Design review of the part built by this model. Coordinates are the model's own, in mm. A direction names the side the tool comes from. Coordinates: 2 decimals unless noted, no trailing zeros. Loops run counter-clockwise (first coordinate to the right, second up) from the corner with the lowest first, then second, coordinate; pieces in that order, holes last. Notation, with made-up numbers: (-33.5, 83) -> (-0.5, 83) arc R26 ccw to (-0.5, 106) -> close; hole circle Ø10 at (10.25, 23.5). An arc over 180 degrees is marked (long way). Use a Markdown table: item, result. Add a question column.
Q1. Take a section at B-B on x = 5. Write out the cut boundary in (y, z).
Q2. Clearance check with a flat-ended pin moving along its axis: pin 1 Ø2 at (x, y) = (134.5, 5) entering from -Z. State where the tip first meets the part, or that it passes through.
Q3. Draft analysis for pull direction Z (two halves, no side actions). For faces 1 (the face through (37, 5, 5)), 2 (the face through (5.766, 4.93, 28.847)), 3 (the face through (84, 5, 160)), state which applies: pulls with the +Z half, pulls with the -Z half, needs draft (parallel to the pull), parting line crosses it, or undercut.
Q4. For faces 4 (the face through (133, 5, 5)), 5 (the face through (84, 10, 79)), 6 (the face through (38.55, 5, 13)), list the 3-axis set-ups (+Z, -Z, +X, -X, +Y, -Y) from which the entire face can be reached by the end or side of a thin tool; tool diameter is ignored.
Q5. Take a section at A-A on z = 27. Write out the cut boundary in (x, y), plus the area to 3 significant figures.
Q6. For probe 1 along Z at (x, y) = (165, 7.5); probe 2 along X at (y, z) = (3.75, 133); probe 3 along X at (y, z) = (9.25, 13.5), list the stretches that pass through material, from the lowest coordinate up.
from build123d import *

# Parameters (mm, degrees)
SKETCH1_W               = 170
SKETCH1_H               = 10
BOSS_EXTRUDE1_DEPTH     = 160
ESQUISSE1_R             = 2
ENL_V_MAT_EXTRU_2_DEPTH = 10
ENL_V_MAT_EXTRU_3_DEPTH = 10


with BuildPart() as part:
    # Sketch1 → Boss-Extrude1 (new body)
    with BuildSketch(Plane.XY):
        with Locations((85, 5)):
            Rectangle(SKETCH1_W, SKETCH1_H)
    extrude(amount=BOSS_EXTRUDE1_DEPTH)

    # Esquisse1 → Enlèv. mat.-Extru.2 (cut)
    with BuildSketch(Plane.XZ):
        with Locations(Location((5, 133, 0), (0, 0, 270))):
            Circle(ESQUISSE1_R)
        with Locations(Location((5, 27, 0), (0, 0, 90))):
            Circle(ESQUISSE1_R)
        with Locations(Location((165, 27, 0), (0, 0, 270))):
            Circle(ESQUISSE1_R)
        with Locations(Location((165, 133, 0), (0, 0, 90))):
            Circle(ESQUISSE1_R)
    extrude(amount=-ENL_V_MAT_EXTRU_2_DEPTH, mode=Mode.SUBTRACT)

    # Esquisse2 → Enlèv. mat.-Extru.3 (cut)
    with BuildSketch(Plane(origin=(0, 0, 0), x_dir=(-1, 0, 0), z_dir=(0, -1, 0))):
        Polygon((-133, -10), (-133, 0), (-137, 0), (-137, -10), (-138.55, -10), (-138.55, -15.5), (-137, -15.5), (-137, -21.5), (-133, -21.5), (-133, -15.5), (-131.45, -15.5), (-131.45, -10), align=None)
        Polygon((-33, -10), (-33, 0), (-37, 0), (-37, -10), (-38.55, -10), (-38.55, -15.5), (-37, -15.5), (-37, -21.5), (-33, -21.5), (-33, -15.5), (-31.45, -15.5), (-31.45, -10), align=None)
    extrude(amount=-ENL_V_MAT_EXTRU_3_DEPTH, mode=Mode.SUBTRACT)


solid = part.part
Answer list:
| question | item | result |
|---|---|---|
| 1 | outline | (0, 0) -> (10, 0) -> (10, 25) -> (0, 25) -> close; (0, 29) -> (10, 29) -> (10, 131) -> (0, 131) -> close; (0, 135) -> (10, 135) -> (10, 160) -> (0, 160) -> close |
| 2 | pin 1 | z = 21.5 |
| 3 | face 1 | needs draft |
| 3 | face 2 | undercut |
| 3 | face 3 | pulls with the +Z half |
| 4 | face 4 | -Z, +Y, -Y |
| 4 | face 5 | +Z, -Z, +X, -X, +Y |
| 4 | face 6 | +Y, -Y |
| 5 | outline | (0, 0) -> (3, 0) -> (3, 10) -> (0, 10) -> close; (7, 0) -> (163, 0) -> (163, 10) -> (7, 10) -> close; (167, 0) -> (170, 0) -> (170, 10) -> (167, 10) -> close |
| 5 | area | 1,620 mm² |
| 6 | probe 1 | 0 to 25, 29 to 131, 135 to 160 |
| 6 | probe 2 | 0 to 3, 7 to 163, 167 to 170 |
| 6 | probe 3 | 0 to 31.45, 38.55 to 131.45, 138.55 to 170 |
